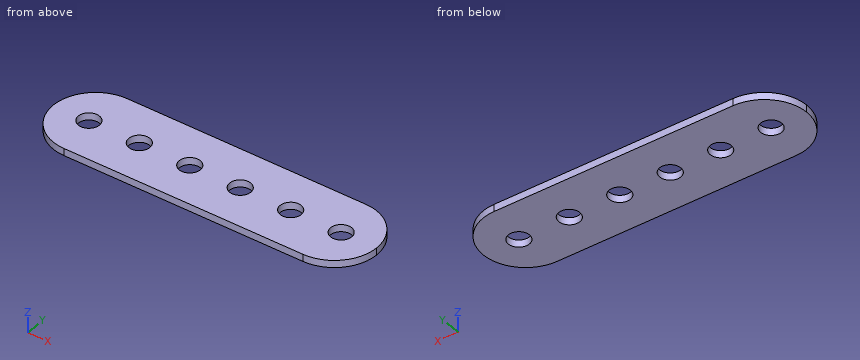
from build123d import *

# Parameters (mm, degrees)
F0_R     = 2.3749
F1_DEPTH = 1.6002


with BuildPart() as f1:
    # F0 (on Top) → F1 (new body)
    with BuildSketch(Plane.XY):
        with BuildLine():
            Line((26.9875, 9.525), (0, 9.525))
            Line((0, 9.525), (-26.9875, 9.525))
            ThreePointArc((-26.9875, 9.525), (-33.722692, 6.735192), (-36.5125, 0))
            ThreePointArc((-36.5125, 0), (-33.722692, -6.735192), (-26.9875, -9.525))
            Line((-26.9875, -9.525), (0, -9.525))
            Line((0, -9.525), (26.9875, -9.525))
            ThreePointArc((26.9875, -9.525), (33.722692, -6.735192), (36.5125, 0))
            ThreePointArc((36.5125, 0), (33.722692, 6.735192), (26.9875, 9.525))
        make_face()
        with Locations((-28.5115, 0)):
            Circle(F0_R, mode=Mode.SUBTRACT)
        with Locations((-17.1069, 0)):
            Circle(F0_R, mode=Mode.SUBTRACT)
        with Locations((-5.7023, 0)):
            Circle(F0_R, mode=Mode.SUBTRACT)
        with Locations((5.7023, 0)):
            Circle(F0_R, mode=Mode.SUBTRACT)
        with Locations((17.1069, 0)):
            Circle(F0_R, mode=Mode.SUBTRACT)
        with Locations((28.5115, 0)):
            Circle(F0_R, mode=Mode.SUBTRACT)
    extrude(amount=F1_DEPTH)


solid = f1.part
The model under review builds one solid part; all positions refer to its coordinate system, in mm. Coordinates: 2 decimals unless noted, no trailing zeros. Loops run counter-clockwise (first coordinate to the right, second up) from the corner with the lowest first, then second, coordinate; pieces in that order, holes last. Notation, with made-up numbers: M 42,-8.5 L 65,-8.5 A3 ccw 65,-4.5 Z; hole C 19.5,-16 d4. An arc over 180 degrees is marked long. Put each result on its own line as item: value. Start each with the question number.
Q1. Add section D-D (y = 6.75). Write out the cut boundary in (x, z).
Q2. Add section C-C (y = -6). Write out the cut boundary in (x, z), and give its area (3 significant figures).
Q3. Wall thickness on line 1 (Y direction, x = 27, z = 0.35) (3 decimals); line 2 (Y direction, x = 29, z = 0.8); line 3 (X direction, y = -8.75, z = 1.4): over which ranges is each line inside the solid? List them lowest first.
Q4. Add section B-B (x = 29). Write out the cut boundary in (y, z).
Q5. Add section A-A (z = 0.5). Count the separate pieces of the cut face and the enclosed holes in it, and give its area (3 significant figures).
Answers:
1. outline: M -33.71,0 L 33.71,0 L 33.71,1.6 L -33.71,1.6 Z
2. outline: M -34.39,0 L 34.39,0 L 34.39,1.6 L -34.39,1.6 Z
2. area: 110 mm^2
3. line 1: y = -9.525 to -1.832, 1.832 to 9.525
3. line 2: y = -9.31 to -2.32, 2.32 to 9.31
3. line 3: x = -30.75 to 30.75
4. outline: M -9.31,0 L -2.32,0 L -2.32,1.6 L -9.31,1.6 Z; M 2.32,0 L 9.31,0 L 9.31,1.6 L 2.32,1.6 Z
5. separate pieces: 1
5. enclosed holes: 6
5. area: 1,210 mm^2
